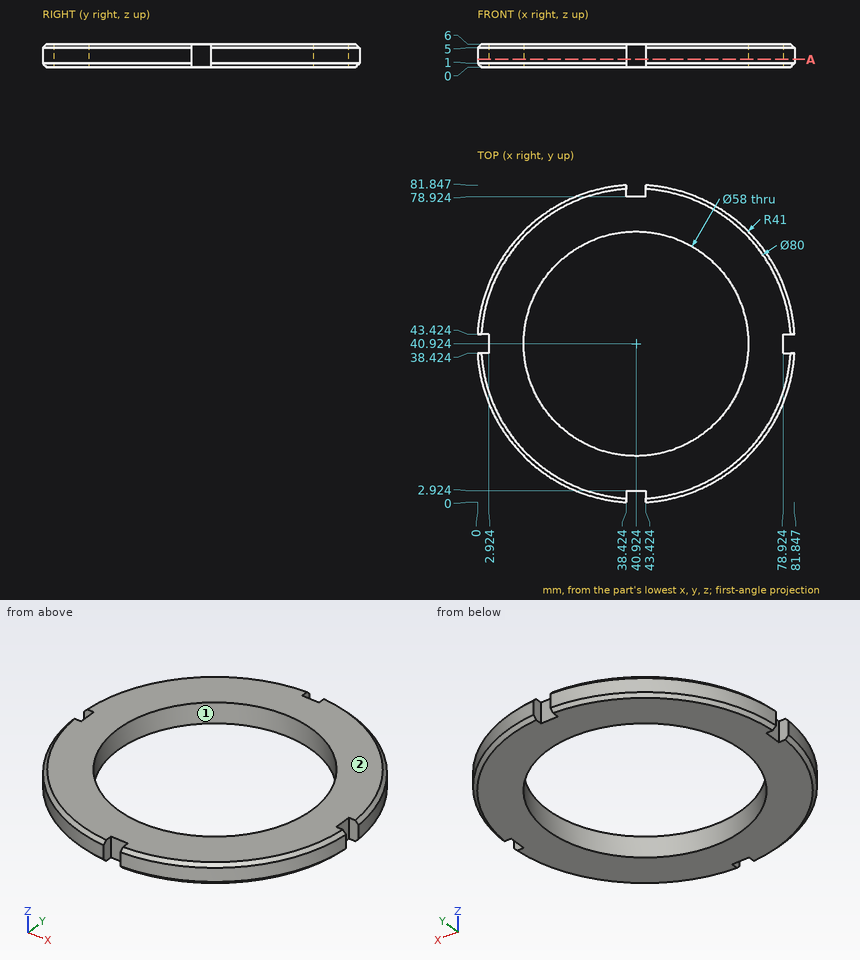
Design review of the part shown in the three views and the two pictorial views. Dimensions are in mm from the part's minimum x, y and z. Give positions to 0.01 mm unless a question says otherwise; leave off trailing zeros. Loops run counter-clockwise (first coordinate to the right, second up) from the corner with the lowest first, then second, coordinate; pieces in that order, holes last. Notation, with made-up numbers: (9.5, 58) -> (27.5, 58) arc R18 ccw to (27.5, 74) -> close; hole circle Ø8 at (58.25, 11). An arc over 180 degrees is marked (long way). Put each result on its own line as item: value. Start each with the question number.
1. Clearance check with flat-ended pins moving along their axes: P1, Ø2.5, axis at y = 79.5, z = 4, coming from the +X side (1 decimal); P2, Ø1.5, axis at y = 49, z = 3.5, coming from the -X side; P3, Ø1.5, axis at y = 15, z = 2.5, coming from the +X side (1 decimal). State where each tip first meets the part, or that it passes through.
2. Mouldability with a two-part tool opening along Y and no side actions: class the marked faces 1 and 2 as released by +Y, released by -Y, zero draft, split by the parting line, or undercut.
3. We need section A-A on z = 2. State the section outline as (x, y) points, then the cut area to 3 significant figures.
4. Wall thickness on probe 1 along X at (y, z) = (64.5, 3.75) (1 decimal); probe 2 along Y at (x, z) = (42, 2.25); probe 3 along X at (y, z) = (59, 1.25) (1 decimal): over which ranges is each line inside the solid? List them lowest first.
Determined:
1. P1: x = 57.9
1. P2: x = 0.58
1. P3: x = 73.3
2. face 1: undercut
2. face 2: zero draft
3. outline: (0, 38.42) arc R41 ccw to (38.42, 0) -> (38.42, 2.92) -> (43.42, 2.92) -> (43.42, 0) arc R41 ccw to (81.85, 38.42) -> (78.92, 38.42) -> (78.92, 43.42) -> (81.85, 43.42) arc R41 ccw to (43.42, 81.85) -> (43.42, 78.92) -> (38.42, 78.92) -> (38.42, 81.85) arc R41 ccw to (0, 43.42) -> (2.92, 43.42) -> (2.92, 38.42) -> close; hole circle Ø58 at (40.92, 40.92)
3. area: 2,580 mm^2
4. probe 1: 7.4 to 24, 57.8 to 74.5
4. probe 2: 2.92 to 11.94, 69.9 to 78.92
4. probe 3: 4.1 to 18.2, 63.6 to 77.7
